Geometry check sheet. Reference: the model listing, model coordinates, mm. A direction names the side the tool comes from. Coordinates: 2 decimals unless noted, no trailing zeros. Order: outer loops, then holes, each group sorted by start corner. A loop starts at its lowest first (then second) coordinate and runs counter-clockwise, first axis right, second up. Notation, with made-up numbers: (82.5, 87.5) - (87.5, 87.5) arc R20 ccw to (87.5, 102.5) - close; hole circle Ø11 at (-15.75, -21). An arc over 180 degrees is marked (long way). Return JSON: item names as keys, results as strings. Group by question number.
Item 1: Section check A-A on y = 37.5. Enter the section's corners in (x, z), then the cut area to 3 significant figures.
Item 2: Section check C-C on y = 14. Enter the section's corners in (x, z).
Item 3: Tool access check on faces 1 (the cylindrical face through (18.1, 15.3, 1.5)), 2 (the cylindrical face through (27.98, 65.4, 1.48)), 3 (the cylindrical face through (63.976, 64.057, 1.479)), 4 (the cylindrical face through (53.399, 68.313, 1.479)). Record the directions out of +Z, -Z, +X, -X, +Y, -Y that give a thin tool (end or side, any length) a straight path to the whole face; none if there is none.
Item 4: Draft check along X on faces 5 (the cylindrical face through (66.424, 31.798, 1.479)), 6 (the cylindrical face through (56.235, 8.324, 1.479)), 7 (the flat face through (37, 30, 3)), 8 (the cylindrical face through (2.866, 35.863, 1.479)). Enter one of: pulls with the +X half, pulls with the -X half, needs draft (parallel to the pull), parting line crosses it, or undercut.
Item 5: Section check D-D on y = 48.5. Enter the section's corners in (x, z).
Item 6: Scan lines: probe 1 along Y at (x, z) = (49.5, 1.85); probe 2 along X at (y, z) = (38, 1.15); probe 3 along X at (y, z) = (14, 1.65). Record each from-to range of solid material in increasing order.
Item 7: Section check B-B on x = 53.5. Enter the section's corners in (y, z), then the cut area to 3 significant figures.
from build123d import *

# Parameters (mm, degrees)
F0_R     = 3
F1_DEPTH = 3
F2_R     = 2
F3_R     = 2


with BuildPart() as f1:
    # F0 (on Top) → F1 (new body)
    with BuildSketch(Plane.XY):
        with BuildLine():
            ThreePointArc((57.514202, 25.269969), (66.546327, 31.896246), (74.956996, 39.295399))
            ThreePointArc((74.956996, 39.295399), (63.695653, 64.333519), (38.3939, 74.989344))
            ThreePointArc((38.3939, 74.989344), (54.563179, 67.459498), (66.146021, 53.895503))
            ThreePointArc((66.146021, 53.895503), (50.919706, 52.664645), (38.084417, 60.947823))
            ThreePointArc((38.084417, 60.947823), (27.82983, 65.456734), (17.216641, 69.041011))
            ThreePointArc((17.216641, 69.041011), (1.163664, 46.769342), (4.586325, 19.529468))
            ThreePointArc((4.586325, 19.529468), (3.022724, 37.297398), (8.978067, 54.11043))
            ThreePointArc((8.978067, 54.11043), (17.657179, 41.539484), (16.901381, 26.282208))
            ThreePointArc((16.901381, 26.282208), (18.123843, 15.14702), (20.326363, 4.163591))
            ThreePointArc((20.326363, 4.163591), (47.640683, 1.397139), (69.519775, 17.981188))
            ThreePointArc((69.519775, 17.981188), (54.914097, 7.743104), (37.375912, 4.494066))
            ThreePointArc((37.375912, 4.494066), (43.923115, 18.295871), (57.514202, 25.269969))
        make_face()
        with Locations((37.5, 37.5)):
            Circle(F0_R, mode=Mode.SUBTRACT)
    extrude(amount=F1_DEPTH)

    # F2
    f2_edges = [f1.edges().sort_by_distance(p)[0] for p in [
        (37.375912, 4.494066, 1.5),
    ]]
    fillet(f2_edges, radius=F2_R)

    # F3
    f3_edges = [f1.edges().sort_by_distance(p)[0] for p in [
        (66.146021, 53.895503, 1.5),
        (8.978067, 54.11043, 1.5),
    ]]
    fillet(f3_edges, radius=F3_R)


solid = f1.part
Computed:
{
 "1": {"outline": "(0, 0) - (3.05, 0) - (3.05, 3) - (0, 3) - close; (18.44, 0) - (34.5, 0) - (34.5, 3) - (18.44, 3) - close; (40.5, 0) - (73.05, 0) - (73.05, 3) - (40.5, 3) - close", "area": "155 mm²"},
 "2": {"outline": "(18.31, 0) - (40.62, 0) - (40.62, 3) - (18.31, 3) - close; (65.3, 0) - (66.72, 0) - (66.72, 3) - (65.3, 3) - close"},
 "3": {"face 1": "+Z, -Z, -Y", "face 2": "+Z, -Z, +Y", "face 3": "+Z, -Z, +X, +Y", "face 4": "+Z, -Z"},
 "4": {"face 5": "pulls with the +X half", "face 6": "undercut", "face 7": "needs draft", "face 8": "undercut"},
 "5": {"outline": "(1.65, 0) - (6.06, 0) - (6.06, 3) - (1.65, 3) - close; (14.38, 0) - (73.35, 0) - (73.35, 3) - (14.38, 3) - close"},
 "6": {"probe 1": "y = 1.97 to 5.89, 22.56 to 53.07, 70.76 to 73.03", "probe 2": "x = 0 to 3.12, 18.38 to 34.54, 40.46 to 73.59", "probe 3": "x = 18.31 to 40.62, 65.3 to 66.72"},
 "7": {"outline": "(3.58, 0) - (7.18, 0) - (7.18, 3) - (3.58, 3) - close; (24.31, 0) - (52.17, 0) - (52.17, 3) - (24.31, 3) - close; (68.24, 0) - (71.42, 0) - (71.42, 3) - (68.24, 3) - close", "area": "104 mm²"}
}
